Input: part model. Units: mm. Frame: model coordinates. A direction names the side the tool comes from. Coordinates: 2 decimals unless noted, no trailing zeros. Order: outer loops, then holes, each group sorted by start corner. A loop starts at its lowest first (then second) coordinate and runs counter-clockwise, first axis right, second up. Notation, with made-up numbers: (-10, 50) -> (-2, 50) arc R26 cw to (-2, 80) -> close; hole circle Ø2 at (4.25, 35.5). An arc over 180 degrees is marked (long way). Use one line per item in the form item = value. Start each with the question number.
1) Section query B-B on y = -1.5. Output: boundary loops of the cut face in (x, z), then the cut area to 3 significant figures.
2) Section query A-A on x = 2.5. Output: boundary loops of the cut face in (y, z).
3) Pin query (flat end, axial travel): pin 1 (1.9 mm diameter, centred on x = -35, y = 30.5, fed in from -Z); pin 2 (2.5 mm diameter, centred on x = -1.5, z = 2.5, fed in from +Y); pin 3 (4 mm diameter, centred on x = 23, z = 2.5, fed in from -Y); pin 4 (4 mm diameter, centred on x = 39, y = -30.5, fed in from +Z). Return the tip coordinate at first contact, or that it passes through.
4) Section query C-C on x = -35. Output: boundary loops of the cut face in (y, z), then the cut area to 3 significant figures.
5) Access query for faces 1 (the flat face through (0, 19.5, 7)), 2 (the flat face through (-20, 4, 6)), 3 (the flat face through (7.5, 10, 0)), 4 (the flat face through (-34, -31.5, -0.5)). Directions: +Z, -Z, +X, -X, +Y, -Y. A direction counts if a zero-diameter tool reaches every point of the face in a straight line with its end or side. Return the directions, or none.
6) Section query D-D on y = -9.5. Output: boundary loops of the cut face in (x, z).
7) Draft query along Y for faces 5 (the flat face through (-1, 0, -1.5)), 6 (the cylindrical face through (-16.467, -14.555, 2.067)), 7 (the cylindrical face through (39.07, -33.25, 0.02)). Return one class per face: pulls with the +Y half, pulls with the -Y half, needs draft (parallel to the pull), parting line crosses it, or undercut.
8) Ray query, line 1 along Y through (x, z) = (-35, -1.3); line 2 along Y through (x, z) = (39, -0.9); line 3 along Y through (x, z) = (14, 2). Return the intervals inside material, ascending.
from build123d import *

# Parameters (mm, degrees)
SKETCH_29_W                          = 90
SKETCH_29_H                          = 61
EXTRUDE_5047_DEPTH                   = 1.5
CUT_EXTRUDE_5288_REACH               = 56.445
SKETCH_30_W                          = 6
SKETCH_30_H                          = 22
FILLET_3_R                           = 3
EXTRUDE_6672_DEPTH                   = 3
CUT_EXTRUDE_7204_REACH               = 58.032
SKETCH_34_R                          = 1.2
SKETCH_35_R                          = 2.25
CUT_EXTRUDE_7829_DEPTH               = 2
FILLET_5_R                           = 2
SKETCH_36_W                          = 40
SKETCH_36_H                          = 39
SKETCH_36_W_2                        = 28.5
SKETCH_36_H_2                        = 28.5
EXTRUDE_8958_DEPTH                   = 12
CHAMFER_2_SIZE                       = 10
CHAMFER_2_SIZE_2                     = 40
CUT_EXTRUDE_9379_REACH               = 60.91
CUT_EXTRUDE_9379_OFFSET_FROM_SURFACE = 1
SKETCH_37_R                          = 0.75
CUT_EXTRUDE_9641_REACH               = 59.172
SKETCH_38_W                          = 15
SKETCH_38_H                          = 8
FILLET_6_R                           = 2
FILLET_7_R                           = 2
FILLET_8_R                           = 3


with BuildPart() as part:
    # Эскиз29 → Extrude 5047 (new, symmetric)
    with BuildSketch(Plane.XY):
        Rectangle(SKETCH_29_W, SKETCH_29_H)
    extrude(amount=EXTRUDE_5047_DEPTH, both=True)

    # Эскиз30 → Cut-Extrude 5288 (cut, up to next)
    with BuildSketch(Plane.XY.offset(1.5), mode=Mode.PRIVATE) as cut_extrude_5288_sk1:
        with Locations((38.5, 6.5)):
            Rectangle(SKETCH_30_W, SKETCH_30_H)
    cut_extrude_5288_tool1 = extrude(cut_extrude_5288_sk1.sketch, amount=-CUT_EXTRUDE_5288_REACH, mode=Mode.PRIVATE) & part.part
    add(cut_extrude_5288_tool1.solids().sort_by_distance((38.5, 6.5, 1.5))[0], mode=Mode.SUBTRACT)

    # Скругление3
    fillet_3_edges = [part.edges().sort_by_distance(p)[0] for p in [
        (-45, 30.5, 0),
        (45, 30.5, 0),
        (45, -30.5, 0),
        (-45, -30.5, 0),
    ]]
    fillet(fillet_3_edges, radius=FILLET_3_R)

    # Эскиз33 → Extrude 6672 (add)
    with BuildSketch(Plane.XY.offset(1.5)):
        with BuildLine():
            Line((-37.75, -30.5), (-32.25, -30.5))
            ThreePointArc((-32.25, -30.5), (-35, -33.25), (-37.75, -30.5))
        make_face()
        with BuildLine():
            Line((-37.75, 30.5), (-32.25, 30.5))
            ThreePointArc((-32.25, 30.5), (-35, 33.25), (-37.75, 30.5))
        make_face()
        with BuildLine():
            Line((41.75, -30.5), (36.25, -30.5))
            ThreePointArc((36.25, -30.5), (39, -33.25), (41.75, -30.5))
        make_face()
        with BuildLine():
            Line((36.25, 30.5), (41.75, 30.5))
            ThreePointArc((41.75, 30.5), (39, 33.25), (36.25, 30.5))
        make_face()
    extrude(amount=-EXTRUDE_6672_DEPTH)

    # Эскиз34 → Cut-Extrude 7204 (cut, up to next)
    with BuildSketch(Plane.XY.offset(1.5), mode=Mode.PRIVATE) as cut_extrude_7204_sk1:
        with Locations((-35, -30.5)):
            Circle(SKETCH_34_R)
    cut_extrude_7204_tool1 = extrude(cut_extrude_7204_sk1.sketch, amount=-CUT_EXTRUDE_7204_REACH, mode=Mode.PRIVATE) & part.part
    # Эскиз34 → Cut-Extrude 7204 (cut, up to next)
    with BuildSketch(Plane.XY.offset(1.5), mode=Mode.PRIVATE) as cut_extrude_7204_sk2:
        with Locations((39, -30.5)):
            Circle(SKETCH_34_R)
    cut_extrude_7204_tool2 = extrude(cut_extrude_7204_sk2.sketch, amount=-CUT_EXTRUDE_7204_REACH, mode=Mode.PRIVATE) & part.part
    # Эскиз34 → Cut-Extrude 7204 (cut, up to next)
    with BuildSketch(Plane.XY.offset(1.5), mode=Mode.PRIVATE) as cut_extrude_7204_sk3:
        with Locations((-35, 30.5)):
            Circle(SKETCH_34_R)
    cut_extrude_7204_tool3 = extrude(cut_extrude_7204_sk3.sketch, amount=-CUT_EXTRUDE_7204_REACH, mode=Mode.PRIVATE) & part.part
    # Эскиз34 → Cut-Extrude 7204 (cut, up to next)
    with BuildSketch(Plane.XY.offset(1.5), mode=Mode.PRIVATE) as cut_extrude_7204_sk4:
        with Locations((39, 30.5)):
            Circle(SKETCH_34_R)
    cut_extrude_7204_tool4 = extrude(cut_extrude_7204_sk4.sketch, amount=-CUT_EXTRUDE_7204_REACH, mode=Mode.PRIVATE) & part.part
    add(cut_extrude_7204_tool1.solids().sort_by_distance((-35, -30.5, 1.5))[0], mode=Mode.SUBTRACT)
    add(cut_extrude_7204_tool2.solids().sort_by_distance((39, -30.5, 1.5))[0], mode=Mode.SUBTRACT)
    add(cut_extrude_7204_tool3.solids().sort_by_distance((-35, 30.5, 1.5))[0], mode=Mode.SUBTRACT)
    add(cut_extrude_7204_tool4.solids().sort_by_distance((39, 30.5, 1.5))[0], mode=Mode.SUBTRACT)

    # Эскиз35 → Cut-Extrude 7829 (cut)
    with BuildSketch(Plane.XY.offset(1.5)):
        with Locations((-35, -30.5)):
            Circle(SKETCH_35_R)
        with Locations((-35, 30.5)):
            Circle(SKETCH_35_R)
        with Locations((39, -30.5)):
            Circle(SKETCH_35_R)
        with Locations((39, 30.5)):
            Circle(SKETCH_35_R)
    extrude(amount=-CUT_EXTRUDE_7829_DEPTH, mode=Mode.SUBTRACT)

    # Скругление5
    fillet_5_edges = [part.edges().sort_by_distance(p)[0] for p in [
        (35.5, -4.5, 0),
        (35.5, 17.5, 0),
        (41.5, 17.5, 0),
        (41.5, -4.5, 0),
    ]]
    fillet(fillet_5_edges, radius=FILLET_5_R)

    # Эскиз36 → Extrude 8958 (add)
    with BuildSketch(Plane.XY.offset(1.5)):
        Rectangle(SKETCH_36_W, SKETCH_36_H)
        Rectangle(SKETCH_36_W_2, SKETCH_36_H_2, mode=Mode.SUBTRACT)
    extrude(amount=EXTRUDE_8958_DEPTH)

    # Фаска2
    # the kernel refuses this chamfer: 40, 10 mm, written as the material it takes off along each edge
    with BuildSketch(Plane(origin=(123.885099991, -19.5, 13.5), x_dir=(0, -0.14778356633657133, -0.9890197255468893), z_dir=(-1, 0, 0))) as chamfer_2_piece_1:
        Polygon((CHAMFER_2_SIZE * 0.989019725547, -CHAMFER_2_SIZE * 0.147783566337), (-CHAMFER_2_SIZE_2 * 0.147783566337, -CHAMFER_2_SIZE_2 * 0.989019725547), (0, 0), align=None)
    extrude(amount=247.770199982, mode=Mode.SUBTRACT)

    # Cut-Extrude 9379: up to this face of the body (flat: up to its plane, moved by the offset)
    cut_extrude_9379_end = Plane(part.part.faces().sort_by_distance((-0.908572553, -0.15524083, -1.5))[0]).offset(-CUT_EXTRUDE_9379_OFFSET_FROM_SURFACE)
    # Эскиз37 → Cut-Extrude 9379 (cut, up to the picked face)
    with BuildSketch(Plane(origin=(0, -1.970588235, 7.882352941), x_dir=(1, 0, 0), z_dir=(0, -0.24253562503633005, 0.9701425001453328)), mode=Mode.PRIVATE) as cut_extrude_9379_sk1:
        with Locations(Location((-16.5, 18.631375785, 0), (0, 0, 270))):
            Circle(SKETCH_37_R)
    cut_extrude_9379_tool1 = split(extrude(cut_extrude_9379_sk1.sketch, amount=-CUT_EXTRUDE_9379_REACH, mode=Mode.PRIVATE), bisect_by=cut_extrude_9379_end, keep=Keep.BOTH, mode=Mode.PRIVATE)
    # Эскиз37 → Cut-Extrude 9379 (cut, up to the picked face)
    with BuildSketch(Plane(origin=(0, -1.970588235, 7.882352941), x_dir=(1, 0, 0), z_dir=(0, -0.24253562503633005, 0.9701425001453328)), mode=Mode.PRIVATE) as cut_extrude_9379_sk2:
        with Locations(Location((16.5, 18.631375785, 0), (0, 0, 270))):
            Circle(SKETCH_37_R)
    cut_extrude_9379_tool2 = split(extrude(cut_extrude_9379_sk2.sketch, amount=-CUT_EXTRUDE_9379_REACH, mode=Mode.PRIVATE), bisect_by=cut_extrude_9379_end, keep=Keep.BOTH, mode=Mode.PRIVATE)
    # Эскиз37 → Cut-Extrude 9379 (cut, up to the picked face)
    with BuildSketch(Plane(origin=(0, -1.970588235, 7.882352941), x_dir=(1, 0, 0), z_dir=(0, -0.24253562503633005, 0.9701425001453328)), mode=Mode.PRIVATE) as cut_extrude_9379_sk3:
        with Locations(Location((16.5, -14.368624215, 0), (0, 0, 270))):
            Circle(SKETCH_37_R)
    cut_extrude_9379_tool3 = split(extrude(cut_extrude_9379_sk3.sketch, amount=-CUT_EXTRUDE_9379_REACH, mode=Mode.PRIVATE), bisect_by=cut_extrude_9379_end, keep=Keep.BOTH, mode=Mode.PRIVATE)
    # Эскиз37 → Cut-Extrude 9379 (cut, up to the picked face)
    with BuildSketch(Plane(origin=(0, -1.970588235, 7.882352941), x_dir=(1, 0, 0), z_dir=(0, -0.24253562503633005, 0.9701425001453328)), mode=Mode.PRIVATE) as cut_extrude_9379_sk4:
        with Locations(Location((-16.5, -14.368624215, 0), (0, 0, 270))):
            Circle(SKETCH_37_R)
    cut_extrude_9379_tool4 = split(extrude(cut_extrude_9379_sk4.sketch, amount=-CUT_EXTRUDE_9379_REACH, mode=Mode.PRIVATE), bisect_by=cut_extrude_9379_end, keep=Keep.BOTH, mode=Mode.PRIVATE)
    add(cut_extrude_9379_tool1.solids().sort_by(Axis((-16.5, 16.104501, 12.401125), (0, 0.24253562503633005, -0.9701425001453328)))[0], mode=Mode.SUBTRACT)
    add(cut_extrude_9379_tool2.solids().sort_by(Axis((16.5, 16.104501, 12.401125), (0, 0.24253562503633005, -0.9701425001453328)))[0], mode=Mode.SUBTRACT)
    add(cut_extrude_9379_tool3.solids().sort_by(Axis((16.5, -15.910201, 4.39745), (0, 0.24253562503633005, -0.9701425001453328)))[0], mode=Mode.SUBTRACT)
    add(cut_extrude_9379_tool4.solids().sort_by(Axis((-16.5, -15.910201, 4.39745), (0, 0.24253562503633005, -0.9701425001453328)))[0], mode=Mode.SUBTRACT)

    # Эскиз38 → Cut-Extrude 9641 (cut, up to next)
    with BuildSketch(Plane.XY.offset(1.5), mode=Mode.PRIVATE) as cut_extrude_9641_sk1:
        with Locations((0, 10.25)):
            Rectangle(SKETCH_38_W, SKETCH_38_H)
    cut_extrude_9641_tool1 = extrude(cut_extrude_9641_sk1.sketch, amount=-CUT_EXTRUDE_9641_REACH, mode=Mode.PRIVATE) & part.part
    add(cut_extrude_9641_tool1.solids().sort_by_distance((0, 10.25, 1.5))[0], mode=Mode.SUBTRACT)

    # Скругление6
    fillet_6_edges = [part.edges().sort_by_distance(p)[0] for p in [
        (-7.5, 6.25, 0),
        (-7.5, 14.25, 0),
        (7.5, 14.25, 0),
        (7.5, 6.25, 0),
    ]]
    fillet(fillet_6_edges, radius=FILLET_6_R)

    # Скругление7
    fillet_7_edges = [part.edges().sort_by_distance(p)[0] for p in [
        (-20, 19.5, 7.375),
        (20, 19.5, 7.375),
        (20, -19.5, 2.5),
        (-20, -19.5, 2.5),
    ]]
    fillet(fillet_7_edges, radius=FILLET_7_R)

    # Скругление8
    fillet_8_edges = [part.edges().sort_by_distance(p)[0] for p in [
        (-37.75, 30.5, 0),
        (-32.25, 30.5, 0),
        (41.75, -30.5, 0),
        (36.25, -30.5, 0),
        (-32.25, -30.5, 0),
        (-37.75, -30.5, 0),
        (36.25, 30.5, 0),
        (41.75, 30.5, 0),
    ]]
    fillet(fillet_8_edges, radius=FILLET_8_R)


solid = part.part
Answers below:
q1.outline = (-45, -1.5) -> (35.5, -1.5) -> (35.5, 1.5) -> (20, 1.5) -> (20, 8) -> (14.25, 8) -> (14.25, 1.5) -> (-14.25, 1.5) -> (-14.25, 8) -> (-20, 8) -> (-20, 1.5) -> (-45, 1.5) -> close; (41.5, -1.5) -> (45, -1.5) -> (45, 1.5) -> (41.5, 1.5) -> close
q1.area = 327 mm^2
q2.outline = (-30.5, -1.5) -> (6.25, -1.5) -> (6.25, 1.5) -> (-14.25, 1.5) -> (-14.25, 4.81) -> (-19.5, 3.5) -> (-19.5, 1.5) -> (-30.5, 1.5) -> close; (14.25, -1.5) -> (30.5, -1.5) -> (30.5, 1.5) -> (19.5, 1.5) -> (19.5, 13.25) -> (14.25, 11.94) -> close
q3.pin_1 = through
q3.pin_2 = 30.5
q3.pin_3 = -30.5
q3.pin_4 = -0.5
q4.outline = (-33.25, -1.5) -> (-31.7, -1.5) -> (-31.7, -0.5) -> (-32.75, -0.5) -> (-32.75, 1.5) -> (-33.25, 1.5) -> close; (-29.3, -1.5) -> (29.3, -1.5) -> (29.3, -0.5) -> (28.25, -0.5) -> (28.25, 1.5) -> (-28.25, 1.5) -> (-28.25, -0.5) -> (-29.3, -0.5) -> close; (31.7, -1.5) -> (33.25, -1.5) -> (33.25, 1.5) -> (32.75, 1.5) -> (32.75, -0.5) -> (31.7, -0.5) -> close
q4.area = 177 mm^2
q5.face_1 = +Z, +X, -X, +Y
q5.face_2 = +Z, -X, +Y, -Y
q5.face_3 = +Z, -Z
q5.face_4 = +Z
q6.outline = (-45, -1.5) -> (45, -1.5) -> (45, 1.5) -> (20, 1.5) -> (20, 6) -> (14.25, 6) -> (14.25, 1.5) -> (-14.25, 1.5) -> (-14.25, 6) -> (-20, 6) -> (-20, 1.5) -> (-45, 1.5) -> close
q7.face_5 = needs draft
q7.face_6 = undercut
q7.face_7 = pulls with the -Y half
q8.line_1 = -33.25 to -31.7, -29.3 to 29.3, 31.7 to 33.25
q8.line_2 = -33.25 to -31.7, -29.3 to -4.5, 17.5 to 29.3, 31.7 to 33.25
q8.line_3 = -19.5 to -14.25, 14.25 to 19.5
